Autodesk Inventor part; units mm, degrees
ref_plane "Work Plane1" through (20.5, 0, 1.5) normal (1, 0, 0) x (0, 0, -1)
ref_plane "YZ Plane" through (0, 0, 0) normal (1, 0, 0) x (0, 1, 0)
ref_plane "XZ Plane" through (0, 0, 0) normal (0, 1, 0) x (-1, 0, 0)
sketch "Sketch1" plane through (0, 0, 0) normal (0, 0, 1) x (1, 0, 0)
  line L0 (0, 0) -> (41, 0)
  line L1 (41, 0) -> (41, 20)
  line L2 (41, 20) -> (0, 20)
  line L3 (0, 20) -> (0, 0)
  dimension "d0" = 41
  dimension "d1" = 20
extrude "Extrusion1" add sketch "Sketch1" along normal blind 1.5
fillet "Fillet1" radius 4 2 edges at (41, 20, 0.75) (0, 20, 0.75)
sketch "Sketch3" plane through (0, 0, 0) normal (0, 0, -1) x (-1, 0, 0)
  line L0 (0, 0) -> (-41, 0)
  line L1 (-41, 0) -> (-39.5, 0)
  line L2 (-39.5, 0) -> (-39.5, 12)
  line L3 (-39.5, 12) -> (-41, 12)
  line L4 (-41, 12) -> (-41, 0)
  dimension "d5" = 1.5
  dimension "d6" = 12
extrude "Extrusion2" add sketch "Sketch3" along normal blind 70
sketch "Sketch4" plane through (0, 0, 0) normal (0, 0, -1) x (-1, 0, 0)
  line L0 (0, 0) -> (-39.5, 0)
  line L1 (0, 0) -> (-1.5, 0)
  line L2 (-1.5, 0) -> (-1.5, 12)
  line L3 (-1.5, 12) -> (0, 12)
  line L4 (0, 12) -> (0, 0)
  dimension "d9" = 1.5
  dimension "d10" = 12
extrude "Extrusion3" add sketch "Sketch4" along normal blind 70
sketch "Sketch5" plane through (0, 0, -70) normal (0, 0, -1) x (-1, 0, 0)
  line L0 (-41, 0) -> (-41, 16)
  line L1 (-41, 0) -> (0, 0)
  line L2 (0, 0) -> (0, 20)
  line L3 (0, 20) -> (-41, 20)
  line L4 (-41, 20) -> (-41, 0)
extrude "Extrusion4" add sketch "Sketch5" along normal blind 1.5
fillet "Fillet2" radius 4 2 edges at (0, 20, -70.75) (41, 20, -70.75)
sketch "Sketch6" plane through (0, 0, 1.5) normal (0, -1, 0) x (1, 0, 0)
  line L0 (4, -73) -> (0, -73)
  line L1 (41, 0) -> (41, -1.5)
  line L2 (0, -73) -> (41, -73)
  line L3 (41, -73) -> (41, 0)
  line L4 (41, 0) -> (0, 0)
  line L5 (0, 0) -> (0, -73)
  point P0 (0, -1.5)
extrude "Extrusion5" add sketch "Sketch6" against normal blind 1.5
ref_plane "Work Plane1" through (20.5, 0, 1.5) normal (1, 0, 0) x (0, 0, -1)
sketch "Sketch9" plane through (20.5, 0, 1.5) normal (1, 0, 0) x (0, 0, -1)
  line L0 (71.5, 1.5) -> (59.5, 1.5)
  line L1 (59.5, 1.5) -> (59.5, 16.5)
  line L2 (59.5, 16.5) -> (71.5, 16.5)
  line L3 (71.5, 16.5) -> (71.5, 1.5)
  point P0 (1.5, 0)
  dimension "d25" = 12
  dimension "d26" = 15
extrude "Extrusion6" add sketch "Sketch9" along normal mid plane 1.5
chamfer "Chamfer1" distance 8 angle 45 1 edges at (20.5, 16.5, -58)
fillet "Fillet3" radius 4 1 edges at (20.5, 16.5, -66)
sketch "Sketch10" plane through (20.5, 0, 1.5) normal (1, 0, 0) x (0, 0, -1)
  line L0 (1.5, 1.5) -> (13.5, 1.5)
  line L1 (13.5, 1.5) -> (13.5, 16.5)
  line L2 (13.5, 16.5) -> (1.5, 16.5)
  line L3 (1.5, 16.5) -> (1.5, 1.5)
  point P0 (1.5, 0)
  dimension "d27" = 12
  dimension "d28" = 15
extrude "Extrusion7" add sketch "Sketch10" along normal mid plane 1.5
chamfer "Chamfer2" distance 8 angle 45 1 edges at (20.5, 16.5, -12)
fillet "Fillet4" radius 4 1 edges at (20.5, 16.5, -4)
sketch "Sketch11" plane through (21.25, 1.5, -12) normal (0, 0, -1) x (-1, 0, 0)
  line L0 (1.5, 7) -> (1.5, 0)
  line L1 (0, 0) -> (1.5, 0)
  line L2 (1.5, 0) -> (1.5, 7)
  line L3 (1.5, 7) -> (0, 7)
  line L4 (0, 7) -> (0, 0)
  point P0 (21.25, -1.5)
extrude "Extrusion8" add sketch "Sketch11" along normal blind 50
fillet "Fillet5" radius 6 2 edges at (20.5, 8.5, -58) (20.5, 8.5, -12)
properties part number "porta pila"
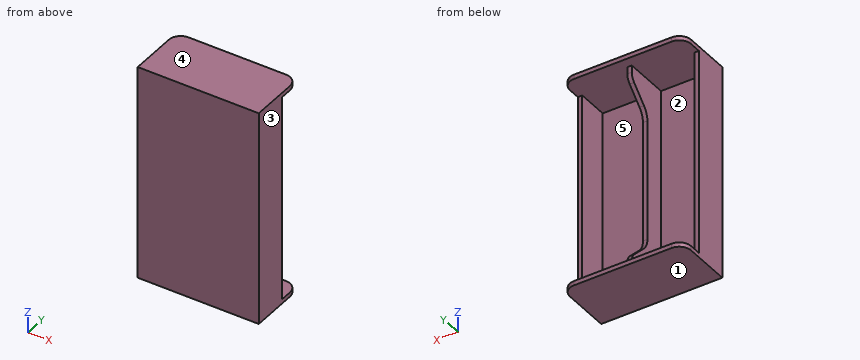
The model under review builds one solid part; all positions refer to its coordinate system, in mm. Face numbers are marked on the shaded views. A direction names the side the tool comes from. Give positions to 0.01 mm unless a question says otherwise; leave off trailing zeros. Write each loop counter-clockwise with the first axis right and the second up, starting at its lowest first coordinate (ties: lowest second). Pieces come first, ordered by that corner, then holes. Notation, with made-up numbers: (17.25, 7.25) -> (71.25, 7.25) arc R9 ccw to (71.25, 23.25) -> close; hole circle Ø10 at (0.5, 28). An arc over 180 degrees is marked (long way). Answer in a Markdown table with one row per item.
1) Add section A-A on x = 25.5. State the section outline as (y, z) points, plus the area to 3 significant figures.
Worked answers:
| item | result |
|---|---|
| outline | (0, -71.5) -> (20, -71.5) -> (20, -70) -> (1.5, -70) -> (1.5, 0) -> (20, 0) -> (20, 1.5) -> (0, 1.5) -> close |
| area | 165 mm² |
2) Add section B-B on y = 3. State the section outline as (x, z) points.
Worked answers:
| item | result |
|---|---|
| outline | (0, -71.5) -> (41, -71.5) -> (41, 1.5) -> (0, 1.5) -> close; hole (1.5, -70) -> (19.75, -70) -> (19.75, 0) -> (1.5, 0) -> close; hole (21.25, -70) -> (39.5, -70) -> (39.5, 0) -> (21.25, 0) -> close |
3) Clearance check with flat-ended pins moving along their axes: P1, Ø5.5, axis at x = 34, z = -29, coming from the +Y side; P2, Ø5, axis at y = 6, z = -20, coming from the -X side; P3, Ø1.2, axis at x = 20.5, z = -26.5, coming from the +Y side; P4, Ø8, axis at y = 17.5, z = -60.5, coming from the -X side. State where each tip first meets the part, or that it passes through.
Worked answers:
| item | result |
|---|---|
| P1 | y = 1.5 |
| P2 | x = 0 |
| P3 | y = 8.5 |
| P4 | through |
4) Mouldability with a two-part tool opening along X and no side actions: class the marked faces 1, 2 and 3 as +X half, -X half, draft (parallel to the pull), parting line (faces both ways), or undercut.
Worked answers:
| item | result |
|---|---|
| face 1 | draft |
| face 2 | undercut |
| face 3 | +X half |
5) For L1, parallel to X at y = 11, z = -2.5; L2, parallel to Z at x = 14, y = 18; L3, parallel to X at y = 11.75, z = -54.5, list the stretches that pass through material, from the lowest coordinate up. Write a range as [from, to].
Worked answers:
| item | result |
|---|---|
| L1 | [0, 1.5], [19.75, 21.25], [39.5, 41] |
| L2 | [-71.5, -70], [0, 1.5] |
| L3 | [0, 1.5], [39.5, 41] |
6) Add section C-C on z = -50. State the section outline as (x, y) points, plus the area to 4 significant figures.
Worked answers:
| item | result |
|---|---|
| outline | (0, 0) -> (41, 0) -> (41, 12) -> (39.5, 12) -> (39.5, 1.5) -> (21.25, 1.5) -> (21.25, 8.5) -> (19.75, 8.5) -> (19.75, 1.5) -> (1.5, 1.5) -> (1.5, 12) -> (0, 12) -> close |
| area | 103.5 mm² |
7) Tool access review of the marked faces 4 and 5: name each direction out of +Z, -Z, +X, -X, +Y, -Y from which nothing blocks a thin tool from reaching the whole face with its end or side.
Worked answers:
| item | result |
|---|---|
| face 4 | +Z, +X, -X, +Y, -Y |
| face 5 | +Y |
8) Add section D-D on z = -66. State the section outline as (x, y) points, plus the area to 3 significant figures.
Worked answers:
| item | result |
|---|---|
| outline | (0, 0) -> (41, 0) -> (41, 12) -> (39.5, 12) -> (39.5, 1.5) -> (21.25, 1.5) -> (21.25, 16.14) -> (19.75, 16.14) -> (19.75, 1.5) -> (1.5, 1.5) -> (1.5, 12) -> (0, 12) -> close |
| area | 115 mm² |
